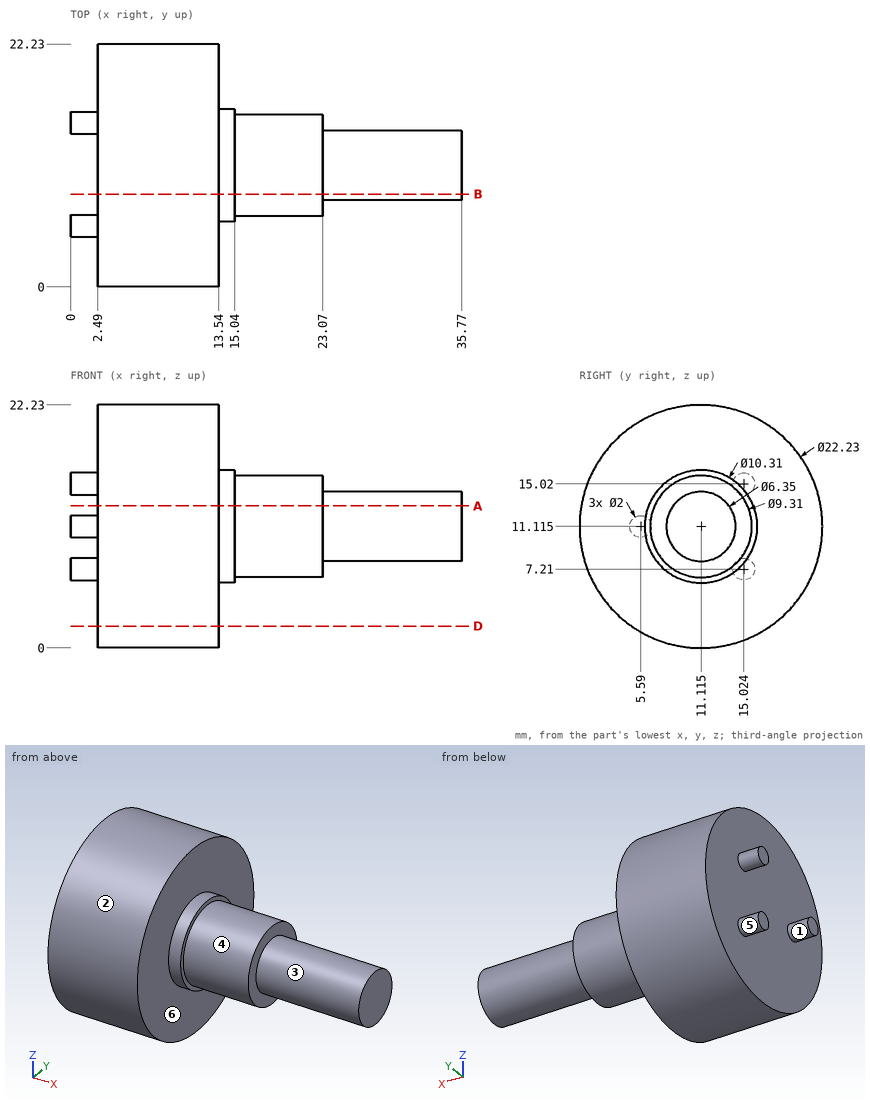
Can you work these out from the drawing? Everything is in mm from the part's minimum corner. A direction names the side the tool comes from. Give positions to 0.01 mm unless a question says otherwise; leave off trailing zeros. Loops run counter-clockwise (first coordinate to the right, second up) from the corner with the lowest first, then second, coordinate; pieces in that order, holes last. Notation, with made-up numbers: (12.5, 58) -> (49.5, 58) arc R19 ccw to (49.5, 75) -> close; hole circle Ø1 at (49.25, 78). An arc over 180 degrees is marked (long way). Return JSON: item names as keys, results as strings.
Item 1: If we section it at A-A on z = 13: List the corners of the cut face in (x, y) for me.
Geometry results:
{"outline": "(2.49, 0.16) -> (13.54, 0.16) -> (13.54, 6.32) -> (15.04, 6.32) -> (15.04, 6.86) -> (23.07, 6.86) -> (23.07, 8.56) -> (35.77, 8.56) -> (35.77, 13.67) -> (23.07, 13.67) -> (23.07, 15.37) -> (15.04, 15.37) -> (15.04, 15.91) -> (13.54, 15.91) -> (13.54, 22.07) -> (2.49, 22.07) -> close"}
Item 2: I need wall thicknesses on L1, parallel to X at y = 4.75, z = 12.75; L2, parallel to X at y = 8, z = 13.5; L3, parallel to Z at x = 5.5, y = 14. Which ranges of each line are inside material? Lowest first, please. Write a range as from..to.
Geometry results:
{"L1": "x = 2.49..13.54", "L2": "x = 2.49..23.07", "L3": "z = 0.38..21.85"}
Item 3: If we section it at B-B on y = 8.5: List the corners of the cut face in (x, z) for me (1 decimal), plus the area to 3 significant figures.
Geometry results:
{"outline": "(2.5, 0.3) -> (13.5, 0.3) -> (13.5, 6.7) -> (15, 6.7) -> (15, 7.3) -> (23.1, 7.3) -> (23.1, 9.3) -> (35.8, 9.3) -> (35.8, 12.9) -> (23.1, 12.9) -> (23.1, 15) -> (15, 15) -> (15, 15.6) -> (13.5, 15.6) -> (13.5, 21.9) -> (2.5, 21.9) -> close", "area": "360 mm²"}
Item 4: I'm going to push flat-ended pins straight in: pin 1 (8 mm diameter, centred on x = 22, y = 18, fed in from +Z); pin 2 (10 mm diameter, centred on x = 29, z = 18, fed in from -Y); pin 3 (4 mm diameter, centred on x = 14, y = 12, fed in from +Z); pin 4 (8 mm diameter, centred on x = 20.5, z = 11, fed in from -Y). Where does each tip first touch, or does it pass through?
Geometry results:
{"pin 1": "stops at z = 14.77", "pin 2": "stops at y = 8.56", "pin 3": "stops at z = 22.23", "pin 4": "stops at y = 6.46"}
Item 5: We'd pull the mould along Z, two halves only. Please class the marked faces 4, 5 and 6: +Z half, -Z half, draft (parallel to the pull), parting line (faces both ways), or undercut.
Geometry results:
{"face 4": "parting line", "face 5": "undercut", "face 6": "draft"}
Item 6: If we section it at D-D on z = 2: List the corners of the cut face in (x, y) for me (1 decimal), plus the area to 3 significant figures.
Geometry results:
{"outline": "(2.5, 4.8) -> (13.5, 4.8) -> (13.5, 17.5) -> (2.5, 17.5) -> close", "area": "141 mm²"}
Item 7: Which directions (+Z, -Z, +X, -X, +Y, -Y) give clear straight access to the entire face, cutting with the end or side of a thin tool? Please do the marked faces 1, 2 and 3.
Geometry results:
{"face 1": "-X", "face 2": "+X, -X", "face 3": "+X"}
